```python
from build123d import *

# Parameters (mm, degrees)
SKETCH_1_R          = 9
EXTRUDE_1_DEPTH     = 5
SKETCH_2_R          = 1.5
CUT_EXTRUDE_1_DEPTH = 10
SKETCH_3_R          = 1.5
CUT_EXTRUDE_2_DEPTH = 10


with BuildPart() as part:
    # 草图1 → 凸台-拉伸1 (new body)
    with BuildSketch(Plane.XY):
        with BuildLine():
            ThreePointArc((-8.629267244, -2.556510674), (-2.479070596, 8.651832695), (8.673703204, 2.401431392))
            add(Edge.make_bspline(
                [(8.673703204, 2.401431392), (7.075929143, 8.172413663), (4.921999012, 15.324710847), (7.430404247, 23.369076832), (8.633989736, 27.459484061)],
                knots=[0, 0, 0, 0, 0.557287964, 1, 1, 1, 1], degree=3))
            ThreePointArc((8.633989736, 27.459484061), (-3.157797251, 21.572170118), (-8.17760204, 33.758566865))
            add(Edge.make_bspline(
                [(-8.17760204, 33.758566865), (-10.239121011, 29.273271712), (-11.449987144, 20.943264961), (-11.113666199, 8.883330205), (-9.769292032, 1.291538409), (-8.629267244, -2.556510674)],
                knots=[0, 0, 0, 0, 0.412769953, 0.64691545, 1, 1, 1, 1], degree=3))
        make_face()
        with Locations((0, 30)):
            Circle(SKETCH_1_R)
        Circle(SKETCH_1_R)
    extrude(amount=EXTRUDE_1_DEPTH)

    # 草图2 → 切除-拉伸1 (cut)
    with BuildSketch(Plane.XY.offset(5)):
        with Locations((0, 30)):
            Circle(SKETCH_2_R)
        Circle(SKETCH_2_R)
    extrude(amount=-CUT_EXTRUDE_1_DEPTH, mode=Mode.SUBTRACT)

    # 草图3 → 切除-拉伸2 (cut)
    with BuildSketch(Plane.XY.offset(5)):
        with Locations((-2.5, 15)):
            Circle(SKETCH_3_R)
    extrude(amount=-CUT_EXTRUDE_2_DEPTH, mode=Mode.SUBTRACT)


solid = part.part
```
Part model, mm, in its own coordinate system. Give positions to 0.01 mm unless a question says otherwise; leave off trailing zeros. Order: outer loops, then holes, each group sorted by start corner. A loop starts at its lowest first (then second) coordinate and runs counter-clockwise, first axis right, second up. Notation, with made-up numbers: M 7.5,30.5 L 37.5,30.5 A31 ccw 37.5,57.5 Z; hole C -38,8 d10. An arc over 180 degrees is marked long. Use a Markdown table: item, result. Add a question column.
(1) Drop flat-ended pins along their axis: P1, Ø1.5, axis at y = -1.5, z = 3.5, coming from the +X side; P2, Ø3, axis at y = 24.5, z = 3, coming from the -X side; P3, Ø3, axis at x = -8, z = 1, coming from the -Y side. Give the stop position or say it passes through.
(2) Probe line 1 along Y through (x, z) = (0, 3.6); line 2 along Y through (x, z) = (-1.25, 0.5); line 3 along Y through (x, z) = (1.25, 1.05). List the from-to ranges inside material, lowest first. Write a range as [from, to].
(3) Saw through at B-B, the plane x = -2.5. Give the cut face in (y, z), and give its area (3 significant figures).
(4) Saw through at D-D, the plane y = -3.5. Give the cut face in (x, z).
(5) Mould opens along Y. For faces 1 (the face through (1, 15, 5)), 2 (the face through (-0.195, 31.487, 2.535)) say: +Y half, -Y half, draft (parallel to the pull), parting line (faces both ways), or undercut.
(6) Saw through at C-C, the plane z = 3.6. Give the number of separate pieces and of enclosed holes in the cut face, and give its area (3 significant figures).
(7) Saw through at A-A, the plane x = 0. Give the cut face in (y, z), and give its area (3 significant figures).
Answer key:
| question | item | result |
|---|---|---|
| 1 | P1 | x = 8.97 |
| 1 | P2 | x = -10.91 |
| 1 | P3 | y = -6.22 |
| 2 | line 1 | [-9, -1.5], [1.5, 28.5], [31.5, 39] |
| 2 | line 2 | [-8.91, -0.83], [0.83, 14.17], [15.83, 29.17], [30.83, 38.91] |
| 2 | line 3 | [-8.91, -0.83], [0.83, 29.17], [30.83, 38.91] |
| 3 | outline | M -8.65,0 L 13.5,0 L 13.5,5 L -8.65,5 Z; M 16.5,0 L 38.65,0 L 38.65,5 L 16.5,5 Z |
| 3 | area | 221 mm^2 |
| 4 | outline | M -8.29,0 L 8.29,0 L 8.29,5 L -8.29,5 Z |
| 5 | face 1 | draft |
| 5 | face 2 | undercut |
| 6 | separate pieces | 1 |
| 6 | enclosed holes | 3 |
| 6 | area | 775 mm^2 |
| 7 | outline | M -9,0 L -1.5,0 L -1.5,5 L -9,5 Z; M 1.5,0 L 28.5,0 L 28.5,5 L 1.5,5 Z; M 31.5,0 L 39,0 L 39,5 L 31.5,5 Z |
| 7 | area | 210 mm^2 |
